Design review of the part built by this model. Coordinates are the model's own, in mm. Face numbers are marked on the shaded views. Give positions to 0.01 mm unless a question says otherwise; leave off trailing zeros. Write each loop counter-clockwise with the first axis right and the second up, starting at its lowest first coordinate (ties: lowest second). Pieces come first, ordered by that corner, then holes. Notation, with made-up numbers: M 34.5,-38.5 L 64.5,-38.5 A17 ccw 64.5,-23.5 Z; hole C 0.5,-14.5 d2. An arc over 180 degrees is marked long. Answer in a Markdown table with one row per item.
```python
from build123d import *

# Parameters (mm, degrees)
SKETCH2_W           = 25.4
SKETCH2_H           = 20.32
SKETCH2_R           = 6.35
SKETCH2_R_2         = 1.778
BOSS_EXTRUDE1_DEPTH = 3.175
SKETCH4_R           = 1.27
CUT_EXTRUDE1_DEPTH  = 3.175


with BuildPart() as part:
    # Sketch2 → Boss-Extrude1 (new body)
    with BuildSketch(Plane.XY):
        with Locations((-1.045882353, 0)):
            Rectangle(SKETCH2_W, SKETCH2_H)
        with Locations((-1.045882353, 0)):
            Circle(SKETCH2_R, mode=Mode.SUBTRACT)
        with Locations((-10.951882353, 0)):
            Circle(SKETCH2_R_2, mode=Mode.SUBTRACT)
        with Locations((8.860117647, 0)):
            Circle(SKETCH2_R_2, mode=Mode.SUBTRACT)
    extrude(amount=BOSS_EXTRUDE1_DEPTH)

    # Sketch4 → Cut-Extrude1 (cut)
    with BuildSketch(Plane.XY.offset(3.175)):
        with Locations((-11.840882353, 8.255)):
            Circle(SKETCH4_R)
        with Locations((-8.792882353, 8.255)):
            Circle(SKETCH4_R)
        with Locations((-5.744882353, 8.255)):
            Circle(SKETCH4_R)
        with Locations((-2.696882353, 8.255)):
            Circle(SKETCH4_R)
        with Locations((0.351117647, 8.255)):
            Circle(SKETCH4_R)
        with Locations((3.399117647, 8.255)):
            Circle(SKETCH4_R)
        with Locations((6.447117647, 8.255)):
            Circle(SKETCH4_R)
        with Locations((9.495117647, 8.255)):
            Circle(SKETCH4_R)
        with Locations((-11.840882353, -8.255)):
            Circle(SKETCH4_R)
        with Locations((-8.792882353, -8.255)):
            Circle(SKETCH4_R)
        with Locations((-5.744882353, -8.255)):
            Circle(SKETCH4_R)
        with Locations((-2.696882353, -8.255)):
            Circle(SKETCH4_R)
        with Locations((0.351117647, -8.255)):
            Circle(SKETCH4_R)
        with Locations((3.399117647, -8.255)):
            Circle(SKETCH4_R)
        with Locations((6.447117647, -8.255)):
            Circle(SKETCH4_R)
        with Locations((9.495117647, -8.255)):
            Circle(SKETCH4_R)
    extrude(amount=-CUT_EXTRUDE1_DEPTH, mode=Mode.SUBTRACT)


solid = part.part
```
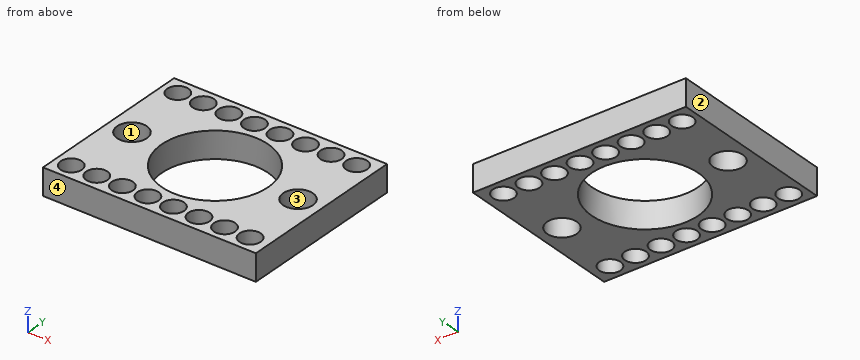
1) Add section A-A (y = 0). Write out the cut boundary in (x, z) (3 decimals).
Geometry says:
| item | result |
|---|---|
| outline | M -13.746,0 L -12.73,0 L -12.73,3.175 L -13.746,3.175 Z; M -9.174,0 L -7.396,0 L -7.396,3.175 L -9.174,3.175 Z; M 5.304,0 L 7.082,0 L 7.082,3.175 L 5.304,3.175 Z; M 10.638,0 L 11.654,0 L 11.654,3.175 L 10.638,3.175 Z |
2) Add section D-D (x = -6). Write out the cut boundary in (y, z) (3 decimals), and give its area (3 significant figures).
Geometry says:
| item | result |
|---|---|
| outline | M -10.16,0 L -9.499,0 L -9.499,3.175 L -10.16,3.175 Z; M -7.011,0 L -3.972,0 L -3.972,3.175 L -7.011,3.175 Z; M 3.972,0 L 7.011,0 L 7.011,3.175 L 3.972,3.175 Z; M 9.499,0 L 10.16,0 L 10.16,3.175 L 9.499,3.175 Z |
| area | 23.5 mm^2 |
3) Add section B-B (z = 2.2). Count the separate pieces of the cut face and the enclosed holes in it, and give its area (3 significant figures).
Geometry says:
| item | result |
|---|---|
| separate pieces | 1 |
| enclosed holes | 19 |
| area | 289 mm^2 |
4) Add section C-C (y = -6). Write out the cut boundary in (x, z) (3 decimals).
Geometry says:
| item | result |
|---|---|
| outline | M -13.746,0 L -3.125,0 L -3.125,3.175 L -13.746,3.175 Z; M 1.033,0 L 11.654,0 L 11.654,3.175 L 1.033,3.175 Z |
5) To check wall thickness, follow probe 1 along X at (y, z) = (1.5, 1.35); probe 2 along Y at (x, z) = (-6.5, 2.6); probe 3 along Y at (x, z) = (-8.75, 2.6). State the ranges of each line that lie inside material, in increasing order. Write a range as [from, to].
Geometry says:
| item | result |
|---|---|
| probe 1 | [-13.75, -11.91], [-10, -7.22], [5.12, 7.91], [9.81, 11.65] |
| probe 2 | [-10.16, -9.28], [-7.23, -3.25], [3.25, 7.23], [9.28, 10.16] |
| probe 3 | [-10.16, -9.52], [-6.99, 6.99], [9.52, 10.16] |
6) The part is to be moulded in two halves that separate along X. For the marked faces 1, 2, 3 and 4, say which applies: released by +X, released by -X, zero draft, split by the parting line, or undercut.
Geometry says:
| item | result |
|---|---|
| face 1 | undercut |
| face 2 | released by -X |
| face 3 | undercut |
| face 4 | zero draft |
